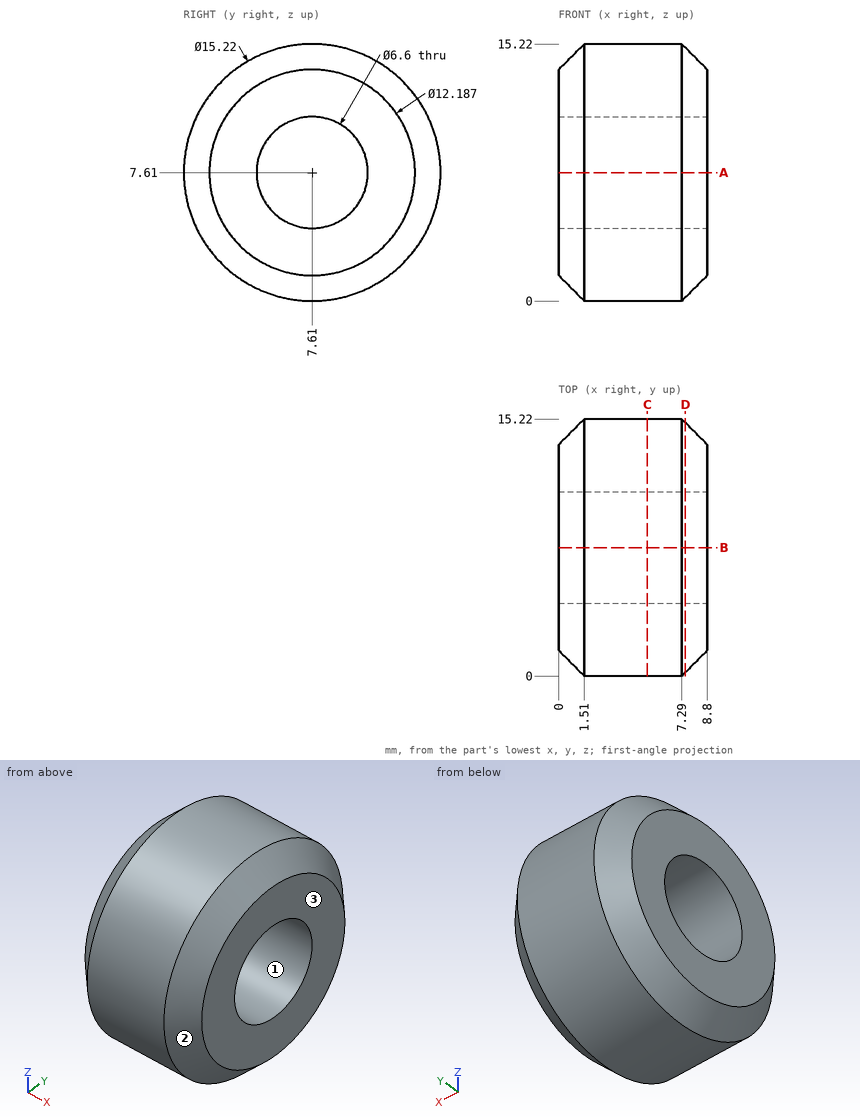
Check sheet for the drawn part. Datum: minimum x, y, z corner. Units: mm. Give positions to 0.01 mm unless a question says otherwise; leave off trailing zeros. Write each loop counter-clockwise with the first axis right and the second up, starting at its lowest first coordinate (ties: lowest second). Pieces come first, ordered by that corner, then holes.
(1) Gauge pin test, flat ends, axial feed: pin 1 (2 mm diameter, centred on x = 2, z = 12.5, fed in from -Y); pin 2 (1.5 mm diameter, centred on x = 2.5, y = 10, fed in from +Z); pin 3 (2 mm diameter, centred on x = 5, z = 6, fed in from +Y). Record the tip position at first contact, or that the pin passes through.
(2) Cross-section at A-A (z = 7.61). Enter the section's corners in (x, y), plus the area to 3 significant figures.
(3) Mould release check, pull along Y, two halves, no side actions. Record for the marked faces 1, 2 and 3: +Y half, -Y half, draft (parallel to the pull), parting line (faces both ways), or undercut.
(4) Cross-section at D-D (x = 7.5). Enter the section's corners in (y, z).
(5) Material ranges on line 1 (Z direction, x = 4, y = 7.61); line 2 (Y direction, x = 2.25, z = 10) (1 decimal); line 3 (Z direction, x = 1.25, y = 9.5) (1 decimal), recorded low to high.
(6) Cross-section at C-C (x = 5.25). Enter the section's corners in (y, z), plus the area to 3 significant figures.
Worked out:
1. pin 1: stops at y = 1.07
1. pin 2: stops at z = 15.04
1. pin 3: stops at y = 15.2
2. outline: (0, 1.52) - (1.51, 0) - (7.29, 0) - (8.8, 1.52) - (8.8, 4.31) - (0, 4.31) - close; (0, 10.91) - (8.8, 10.91) - (8.8, 13.7) - (7.29, 15.22) - (1.51, 15.22) - (0, 13.7) - close
2. area: 71.3 mm2
3. face 1: undercut
3. face 2: parting line
3. face 3: draft
4. outline: circle Ø14.8 at (7.61, 7.61); hole circle Ø6.6 at (7.61, 7.61)
5. line 1: z = 0 to 4.31, 10.91 to 15.22
5. line 2: y = 0.4 to 5.3, 9.9 to 14.8
5. line 3: z = 0.5 to 4.9, 10.3 to 14.7
6. outline: circle Ø15.22 at (7.61, 7.61); hole circle Ø6.6 at (7.61, 7.61)
6. area: 148 mm2
